Answer from the drawing. Dimensions are ordinates in mm from the lowest x, y and z of the part. A direction names the side the tool comes from. Give positions to 0.01 mm unless a question says otherwise; leave off trailing zeros. Loops run counter-clockwise (first coordinate to the right, second up) from the corner with the lowest first, then second, coordinate; pieces in that order, holes last.
(1) Find section A-A, the plane z = 9.5. Write down the section's boundary in (x, y), then the cut area to 3 significant figures.
(2) Straight lines are drawn through the part: probe 1 along Z at (x, y) = (22.5, 20); probe 2 along Y at (x, z) = (7, 3.1); probe 3 along X at (y, z) = (9.5, 2.25). For each, find the intervals that lie inside material, in ascending order.
(3) Find section B-B, the plane z = 4.5. Write down the section's boundary in (x, y).
(4) Determine the mould class of the marked faces 3, 4 and 5 for opening direction Y: pulls with the +Y half, pulls with the -Y half, needs draft (parallel to the pull), parting line crosses it, or undercut.
(5) Which of the six approach directions +Z, -Z, +X, -X, +Y, -Y give full straight-line access (tool end or side, diameter ignored) to the marked faces 1 and 2?
(6) Find section C-C, the plane x = 20. Write down the section's boundary in (y, z), then the cut area to 3 significant figures.
(7) Each of these flat-tipped pins is pushed along its axis until it touches: P1, Ø1, axis at x = 23, z = 10.5, coming from the +Y side; P2, Ø8, axis at x = 21, z = 6.5, coming from the -Y side; P3, Ø8, axis at y = 15, z = 2, coming from the +X side (3 decimals). Where does it stop, or does it pass through?
(8) Find section D-D, the plane z = 12.5. Write down the section's boundary in (x, y), then the cut area to 3 significant figures.
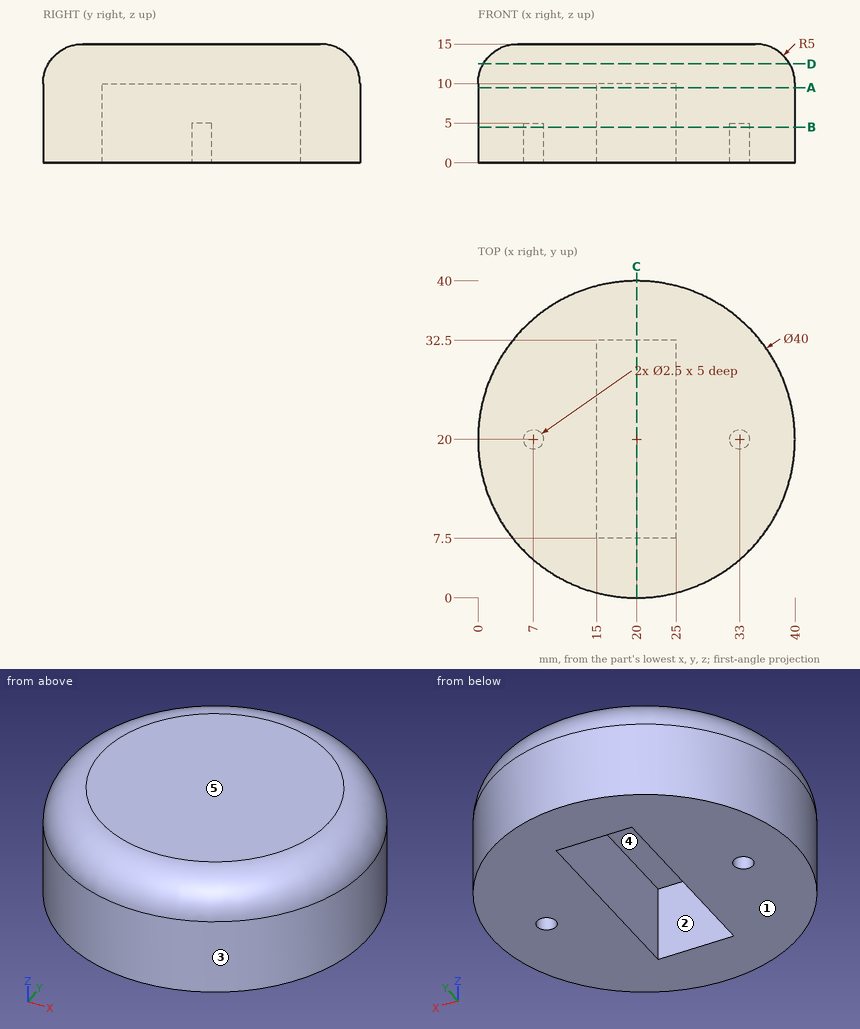
Entries:
1. outline: circle Ø40 at (20, 20); hole (15, 7.5) - (25, 7.5) - (25, 32.5) - (15, 32.5) - close
1. area: 1,010 mm2
2. probe 1: z = 10 to 15
2. probe 2: y = 4.8 to 18.75, 21.25 to 35.2
2. probe 3: x = 2.98 to 15, 25 to 37.02
3. outline: circle Ø40 at (20, 20); hole circle Ø2.5 at (7, 20); hole (15, 7.5) - (25, 7.5) - (25, 32.5) - (15, 32.5) - close; hole circle Ø2.5 at (33, 20)
4. face 3: parting line crosses it
4. face 4: undercut
4. face 5: needs draft
5. face 1: -Z, +X, -X, +Y, -Y
5. face 2: -Z
6. outline: (0, 0) - (7.5, 0) - (7.5, 10) - (32.5, 10) - (32.5, 0) - (40, 0) - (40, 10) arc R5 ccw to (35, 15) - (5, 15) arc R5 ccw to (0, 10) - close
6. area: 339 mm2
7. P1: stops at y = 39.83
7. P2: stops at y = 0
7. P3: stops at x = 39.975
8. outline: circle Ø38.66 at (20, 20)
8. area: 1,170 mm2
